Study the drawing (mm; zero at the part's minimum x, y, z) and answer. A direction names the side the tool comes from. Round coordinates to 2 decimals unless told otherwise and drop trailing zeros. Loops run counter-clockwise (first coordinate to the right, second up) from the corner with the lowest first, then second, coordinate; pieces in that order, holes last. Notation, with made-up numbers: (-38.5, 66.25) -> (-5.5, 66.25) arc R22 ccw to (-5.5, 85.25) -> close; hole circle Ø3 at (-37.5, 85.25). An arc over 180 degrees is marked (long way). Answer in a Markdown table with one row per item. Add a question column.
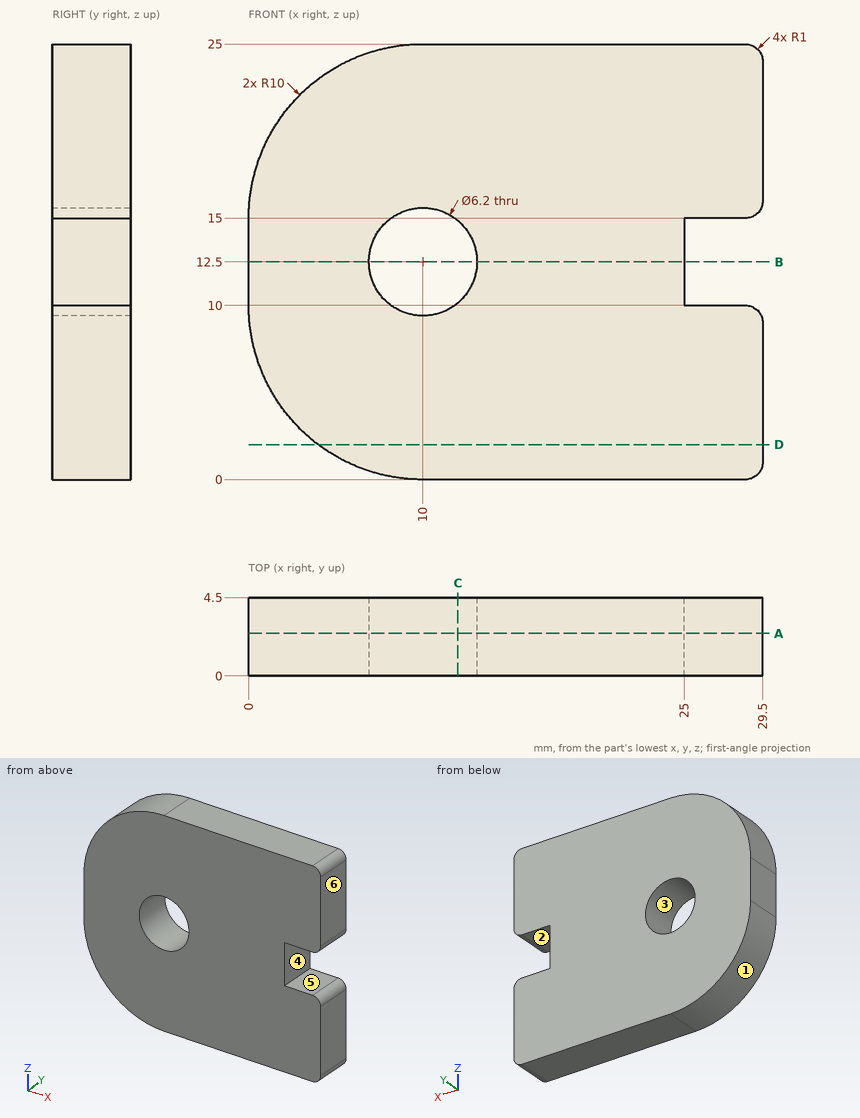
Item 1: Section A-A, the plane y = 2.45 is taken. Write down the section's boundary in (x, z), and give its area (3 significant figures).
Item 2: Section D-D, the plane z = 2 is taken. Write down the section's boundary in (x, y).
Item 3: Section B-B, the plane z = 12.5 is taken. Write down the section's boundary in (x, y), and give its area (3 significant figures).
Item 4: A flat-ended cylindrical pin translates along its axis: P1, Ø4, axis at x = 5.5, z = 8.5, coming from the -Y side. Find the tip coordinate at first contact, or state that the pin passes through.
Item 5: Consider L1, parallel to X at y = 0.9, z = 12.5; L2, parallel to Z at x = 11.75, y = 3.5; L3, parallel to X at y = 1.6, z = 14. Determine where each line is inside the solid, lowest interval first. Write a range as from..to.
Item 6: Section C-C, the plane x = 12 is taken. Write down the section's boundary in (y, z), and give its area (3 significant figures).
Item 7: For the marked faces 5 and 6, determine the directions among +Z, -Z, +X, -X, +Y, -Y from which every point of the face is accessible in a straight line to the end or side of a thin tool.
Item 8: The mould has two halves that part along X. Classify the marked faces 1, 2, 3 and 4: +X half, -X half, draft (parallel to the pull), parting line (faces both ways), or undercut.
Here are the results:
| question | item | result |
|---|---|---|
| 1 | outline | (0, 10) arc R10 ccw to (10, 0) -> (28.5, 0) arc R1 ccw to (29.5, 1) -> (29.5, 9) arc R1 ccw to (28.5, 10) -> (25, 10) -> (25, 15) -> (28.5, 15) arc R1 ccw to (29.5, 16) -> (29.5, 24) arc R1 ccw to (28.5, 25) -> (10, 25) arc R10 ccw to (0, 15) -> close; hole circle Ø6.2 at (10, 12.5) |
| 1 | area | 641 mm² |
| 2 | outline | (4, 0) -> (29.5, 0) -> (29.5, 4.5) -> (4, 4.5) -> close |
| 3 | outline | (0, 0) -> (6.9, 0) -> (6.9, 4.5) -> (0, 4.5) -> close; (13.1, 0) -> (25, 0) -> (25, 4.5) -> (13.1, 4.5) -> close |
| 3 | area | 84.6 mm² |
| 4 | P1 | stops at y = 0 |
| 5 | L1 | x = 0..6.9, 13.1..25 |
| 5 | L2 | z = 0..9.94, 15.06..25 |
| 5 | L3 | x = 0..7.29, 12.71..25 |
| 6 | outline | (0, 0) -> (4.5, 0) -> (4.5, 10.13) -> (0, 10.13) -> close; (0, 14.87) -> (4.5, 14.87) -> (4.5, 25) -> (0, 25) -> close |
| 6 | area | 91.2 mm² |
| 7 | face 5 | +X, +Y, -Y |
| 7 | face 6 | +Z, -Z, +X, +Y, -Y |
| 8 | face 1 | -X half |
| 8 | face 2 | draft |
| 8 | face 3 | undercut |
| 8 | face 4 | +X half |
